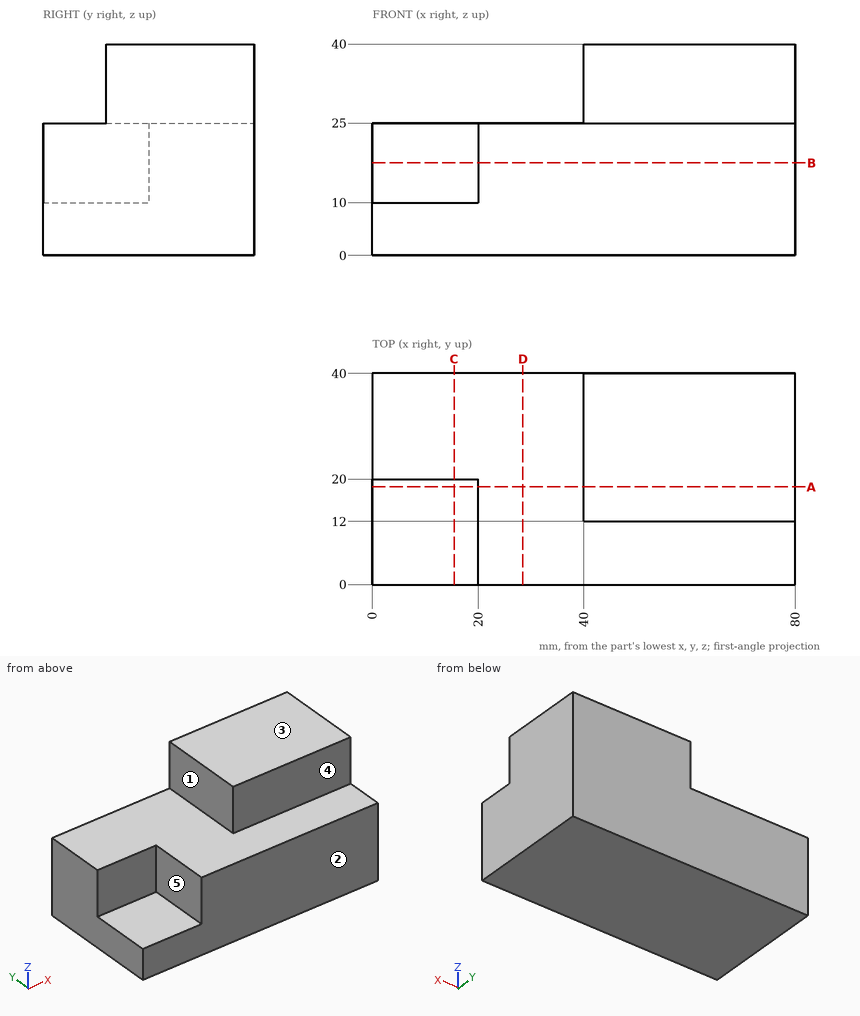
Source: three-view drawing plus pictorial views. Frame: mm from the lowest corner of the part. A direction names the side the tool comes from. Give positions to 0.01 mm unless a question says otherwise; leave off trailing zeros. Order: outer loops, then holes, each group sorted by start corner. A loop starts at its lowest first (then second) coordinate and runs counter-clockwise, first axis right, second up. Notation, with made-up numbers: (62.5, 54) - (114.5, 54) arc R20 ccw to (114.5, 86) - close; hole circle Ø10 at (33.25, 43). An arc over 180 degrees is marked (long way). Put each result on its own line as item: value.
Item 1: Contact query for flat-ended pins moving along their axis: pin 1 (12 mm diameter, centred on x = 14, z = 14, fed in from -Y); pin 2 (8 mm diameter, centred on x = 24, z = 30, fed in from +Y); pin 3 (22 mm diameter, centred on x = 11, y = 14.5, fed in from +Z); pin 4 (4 mm diameter, centred on x = 71.5, z = 32, fed in from -Y). Output: stop coordinate, or through.
Found:
pin 1: stops at y = 0
pin 2: passes through
pin 3: stops at z = 25
pin 4: stops at y = 12
Item 2: Section query D-D, the plane x = 28.5. Return loops of the section in (y, z), then the cut area to 3 significant figures.
Found:
outline: (0, 0) - (40, 0) - (40, 25) - (0, 25) - close
area: 1,000 mm^2
Item 3: Ray query, L1, parallel to Z at x = 31.5, y = 33.5; L2, parallel to X at y = 2, z = 12.5; L3, parallel to Y at x = 58, z = 31.5. Return the intervals inside material, ascending. Write a range as from..to.
Found:
L1: z = 0..25
L2: x = 20..80
L3: y = 12..40
Item 4: Section query C-C, the plane x = 15.5. Return loops of the section in (y, z).
Found:
outline: (0, 0) - (40, 0) - (40, 25) - (20, 25) - (20, 10) - (0, 10) - close
Item 5: Section query A-A, the plane y = 18.5. Return loops of the section in (x, z), then the cut area to 3 significant figures.
Found:
outline: (0, 0) - (80, 0) - (80, 40) - (40, 40) - (40, 25) - (20, 25) - (20, 10) - (0, 10) - close
area: 2,300 mm^2
Item 6: Section query B-B, the plane z = 17.5. Return loops of the section in (x, y).
Found:
outline: (0, 20) - (20, 20) - (20, 0) - (80, 0) - (80, 40) - (0, 40) - close
Item 7: Access query for the marked faces 1, 2, 3, 4 and 5. Directions: +Z, -Z, +X, -X, +Y, -Y. A direction counts if a zero-diameter tool reaches every point of the face in a straight line with its end or side. Return the directions, or none.
Found:
face 1: +Z, -X, +Y, -Y
face 2: +Z, -Z, +X, -X, -Y
face 3: +Z, +X, -X, +Y, -Y
face 4: +Z, +X, -X, -Y
face 5: +Z, -X, -Y
